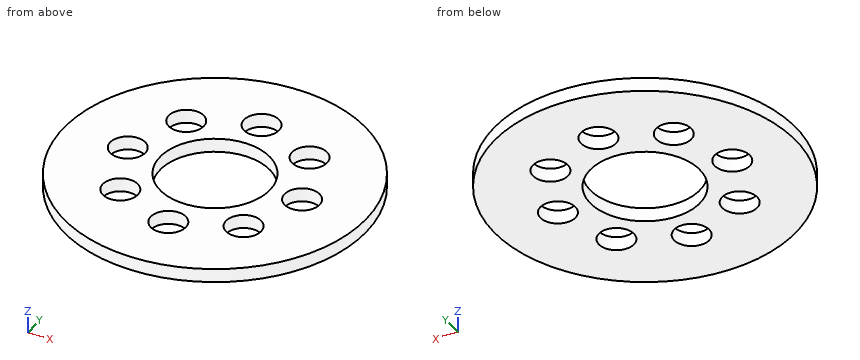
```python
from build123d import *

# Parameters (mm, degrees)
F0_R     = 34.925
F0_R_2   = 4.064
F0_R_3   = 12.7
F1_DEPTH = 3.175


with BuildPart() as f1:
    # F0 (on Top) → F1 (new body)
    with BuildSketch(Plane.XY):
        Circle(F0_R)
        with Locations((-14.188805, -14.188805)):
            Circle(F0_R_2, mode=Mode.SUBTRACT)
        with Locations((0, -20.066)):
            Circle(F0_R_2, mode=Mode.SUBTRACT)
        with Locations((14.188805, -14.188805)):
            Circle(F0_R_2, mode=Mode.SUBTRACT)
        with Locations((-20.066, 0)):
            Circle(F0_R_2, mode=Mode.SUBTRACT)
        with Locations((-14.188805, 14.188805)):
            Circle(F0_R_2, mode=Mode.SUBTRACT)
        Circle(F0_R_3, mode=Mode.SUBTRACT)
        with Locations((14.188805, 14.188805)):
            Circle(F0_R_2, mode=Mode.SUBTRACT)
        with Locations((20.066, 0)):
            Circle(F0_R_2, mode=Mode.SUBTRACT)
        with Locations((0, 20.066)):
            Circle(F0_R_2, mode=Mode.SUBTRACT)
    extrude(amount=F1_DEPTH)


solid = f1.part
```
Read the model definition and answer for the solid it produces. Units are mm, in the model's axes. Give positions to 0.01 mm unless a question says otherwise; leave off trailing zeros. Write each loop counter-clockwise with the first axis right and the second up, starting at its lowest first coordinate (ties: lowest second). Pieces come first, ordered by that corner, then holes. Notation, with made-up numbers: (72.5, -32.75) -> (76.5, -32.75) arc R33 ccw to (76.5, 6.25) -> close; hole circle Ø4 at (31, 23.25). An arc over 180 degrees is marked (long way). Answer in a Markdown table with one row per item.
1) Each of these flat-tipped pins is pushed along its axis until it touches: pin 1 Ø6.5 at (x, y) = (14.19, 14.19) entering from -Z; pin 2 Ø1 at (x, z) = (9.5, 2.5) entering from -Y; pin 3 Ø1 at (x, z) = (4.5, 2.5) entering from -Y. Where does it stop, or does it pass through?
Results list:
| item | result |
|---|---|
| pin 1 | through |
| pin 2 | y = -33.75 |
| pin 3 | y = -34.7 |
2) Section A-A on x = 0 is taken. Give the vertices of the cut face in (y, z) (3 decimals).
Results list:
| item | result |
|---|---|
| outline | (-34.925, 0) -> (-24.13, 0) -> (-24.13, 3.175) -> (-34.925, 3.175) -> close; (-16.002, 0) -> (-12.7, 0) -> (-12.7, 3.175) -> (-16.002, 3.175) -> close; (12.7, 0) -> (16.002, 0) -> (16.002, 3.175) -> (12.7, 3.175) -> close; (24.13, 0) -> (34.925, 0) -> (34.925, 3.175) -> (24.13, 3.175) -> close |
3) Section C-C on z = 0.7 is taken. Count the separate pieces of the cut face and the enclosed holes in it, plus the area to 3 significant figures.
Results list:
| item | result |
|---|---|
| separate pieces | 1 |
| enclosed holes | 9 |
| area | 2,910 mm^2 |
4) Straight lines are drawn through the part: line 1 (Y direction, x = 0, z = 0.9) (3 decimals); line 2 (Y direction, x = -15, z = 1.4); line 3 (Y direction, x = -2.5, z = 1.2). For each, find the intervals that lie inside material, in ascending order. Write a range as [from, to].
Results list:
| item | result |
|---|---|
| line 1 | [-34.925, -24.13], [-16.002, -12.7], [12.7, 16.002], [24.13, 34.925] |
| line 2 | [-31.54, -18.17], [-10.21, 10.21], [18.17, 31.54] |
| line 3 | [-34.84, -23.27], [-16.86, -12.45], [12.45, 16.86], [23.27, 34.84] |
5) Section D-D on x = -25.5 is taken. Give the vertices of the cut face in (y, z) (3 decimals).
Results list:
| item | result |
|---|---|
| outline | (-23.864, 0) -> (23.864, 0) -> (23.864, 3.175) -> (-23.864, 3.175) -> close |
